Here's how the part is built. I have some questions about the finished solid (model axes, mm). A direction names the side the tool comes from. Round coordinates to 2 decimals unless told otherwise and drop trailing zeros. Write each loop counter-clockwise with the first axis right and the second up, starting at its lowest first coordinate (ties: lowest second). Pieces come first, ordered by that corner, then holes. Notation, with made-up numbers: (80, -32) - (115, -32) arc R18 cw to (115, -11) - close; hole circle Ø9 at (75, 58). An arc over 180 degrees is marked (long way). One line per item, written item: value. Start each with the question number.
Item 1: If I drill on line 1 (Z direction, x = 0, y = -14.5); line 2 (Z direction, x = 0, y = -3.25) (1 decimal); line 3 (X direction, y = -18.5, z = 0.25), over which ranges is the centre line in solid material (lowest first)?
Item 2: Imagine slicing it at B-B, the plane z = 0. Please give me the cut outline in (x, y) (1 decimal).
Item 3: Imagine slicing it at C-C, the plane y = -9.5. Please give me the cut outline in (x, z) (1 decimal).
Item 4: Imagine slicing it at D-D, the plane z = -3.5. Please give me the cut outline in (x, y) (1 decimal).
Item 5: Thinking about a two-plate mould opening in X: for faces 1 (the face through (1, -1.27, 8)), 2 (the face through (-7.559, -2.209, -5.796)), 3 (the face through (-0.69, -3.91, -3.1)), which applies, released by +X, released by -X, zero draft, split by the parting line, or undercut?
Item 6: For P1, Ø10, axis at y = -22, z = -1, coming from the +X side; P2, Ø8, axis at y = -17, z = 3, coming from the -X side; P3, Ø8, axis at x = 0, z = -3.5, coming from the +Y side; P4, Ø1.9, axis at x = 1.5, z = 0, coming from the +Y side, each with a flat end and sliding along its axis, tell me the tip position at first contact or that it passes through.
Item 7: Imagine slicing it at A-A, the plane x = 0. Please give me the cut outline in (y, z) (1 decimal), then the cut area to 3 significant figures.
Item 8: For faces 4 (the face through (5.3, -21.49, 1.67)), 5 (the face through (3, 0, -2)), 6 (the face through (7.16, -0.63, 2.25)), which set-ups out of +Z, -Z, +X, -X, +Y, -Y let a thin tool reach every point of the face, with its end or its side?
```python
from build123d import *

# Parameters (mm, degrees)
F0_R     = 9.525
F0_R_2   = 7.5057
F0_R_3   = 3.175
F1_DEPTH = 25.4
F2_R     = 5.55625
F3_DEPTH = 7.9375
F2_R_2   = 9.525
F2_R_3   = 7.9375
F5_DEPTH = 22.225
F6_DEPTH = 1.27
F7_DEPTH = 7.9375
F8_D     = 5.1054


with BuildPart() as f1:
    # F0 (on Front) → F1 (new body)
    with BuildSketch(Plane.XZ):
        Circle(F0_R)
        Circle(F0_R_2, mode=Mode.SUBTRACT)
        Circle(F0_R_2)
        Circle(F0_R_3, mode=Mode.SUBTRACT)
        Circle(F0_R_3)
    extrude(amount=F1_DEPTH)

    # F2 (on face) → F3 (cut)
    with BuildSketch(Plane.XZ.offset(25.4)):
        Circle(F2_R)
    extrude(amount=-F3_DEPTH, mode=Mode.SUBTRACT)

    # F2 (on face) → F5 (cut)
    with BuildSketch(Plane.XZ.offset(25.4)):
        Circle(F2_R_2)
        Circle(F2_R_3, mode=Mode.SUBTRACT)
    extrude(amount=-F5_DEPTH, mode=Mode.SUBTRACT)

    # F0 (on Front) → F6 (cut)
    with BuildSketch(Plane.XZ):
        Circle(F0_R)
        Circle(F0_R_2, mode=Mode.SUBTRACT)
    extrude(amount=F6_DEPTH, mode=Mode.SUBTRACT)

    # F0 (on Front) → F7 (cut)
    with BuildSketch(Plane.XZ):
        Circle(F0_R_3)
    extrude(amount=F7_DEPTH, mode=Mode.SUBTRACT)

    # F8 (through all)
    with Locations(Plane.XZ.offset(17.4625)):
        with Locations((0, 0)):
            Hole(F8_D / 2)


solid = f1.part
```
Values follow:
1. line 1: z = -7.94 to -2.55, 2.55 to 7.94
1. line 2: z = -7.9 to -3.2, 3.2 to 7.9
1. line 3: x = -7.93 to -5.55, 5.55 to 7.93
2. outline: (-9.5, -3.2) - (-7.9, -3.2) - (-7.9, -25.4) - (-5.6, -25.4) - (-5.6, -17.5) - (-2.6, -17.5) - (-2.6, -7.9) - (-3.2, -7.9) - (-3.2, 0) - (-7.5, 0) - (-7.5, -1.3) - (-9.5, -1.3) - close; (2.6, -17.5) - (5.6, -17.5) - (5.6, -25.4) - (7.9, -25.4) - (7.9, -3.2) - (9.5, -3.2) - (9.5, -1.3) - (7.5, -1.3) - (7.5, 0) - (3.2, 0) - (3.2, -7.9) - (2.6, -7.9) - close
3. outline: circle Ø15.9 at (0, 0); hole circle Ø5.1 at (0, 0)
4. outline: (-8.9, -3.2) - (-7.1, -3.2) - (-7.1, -25.4) - (-4.3, -25.4) - (-4.3, -17.5) - (4.3, -17.5) - (4.3, -25.4) - (7.1, -25.4) - (7.1, -3.2) - (8.9, -3.2) - (8.9, -1.3) - (6.6, -1.3) - (6.6, 0) - (-6.6, 0) - (-6.6, -1.3) - (-8.9, -1.3) - close
5. face 1: zero draft
5. face 2: split by the parting line
5. face 3: undercut
6. P1: stops at x = 7.94
6. P2: stops at x = -7.94
6. P3: stops at y = 0
6. P4: passes through
7. outline: (-25.4, -7.9) - (-3.2, -7.9) - (-3.2, -9.5) - (-1.3, -9.5) - (-1.3, -7.5) - (0, -7.5) - (0, -3.2) - (-7.9, -3.2) - (-7.9, -2.6) - (-17.5, -2.6) - (-17.5, -5.6) - (-25.4, -5.6) - close; (-25.4, 5.6) - (-17.5, 5.6) - (-17.5, 2.6) - (-7.9, 2.6) - (-7.9, 3.2) - (0, 3.2) - (0, 7.5) - (-1.3, 7.5) - (-1.3, 9.5) - (-3.2, 9.5) - (-3.2, 7.9) - (-25.4, 7.9) - close
7. area: 221 mm^2
8. face 4: -Y
8. face 5: +Z, -Z, +X, -X, +Y
8. face 6: +Y
